from build123d import *

# Parameters (mm, degrees)
SKETCH2_R           = 13.75
BOSS_EXTRUDE1_DEPTH = 26.5
SKETCH3_R           = 2
BOSS_EXTRUDE2_DEPTH = 3.5
SKETCH4_R           = 1.25
CUT_EXTRUDE1_DEPTH  = 5
BOSS_EXTRUDE3_REACH = 39.959
SKETCH1_R           = 2
SKETCH5_R           = 1.25
CUT_EXTRUDE2_DEPTH  = 5


with BuildPart() as part:
    # Sketch2 → Boss-Extrude1 (new body)
    with BuildSketch(Plane(origin=(0, 2.6, 0), x_dir=(1, 0, 0), z_dir=(0, 1, 0))):
        with Locations(Location((0, 0, 0), (0, 0, 270))):
            Circle(SKETCH2_R)
    extrude(amount=BOSS_EXTRUDE1_DEPTH)

    # Sketch3 → Boss-Extrude2 (add)
    with BuildSketch(Plane(origin=(0, 29.1, 0), x_dir=(1, 0, 0), z_dir=(0, 1, 0))):
        with Locations(Location((0, 0, 0), (0, 0, 270))):
            Circle(SKETCH3_R)
    extrude(amount=BOSS_EXTRUDE2_DEPTH)

    # Sketch4 → Cut-Extrude1 (cut)
    with BuildSketch(Plane(origin=(0, 29.1, 0), x_dir=(1, 0, 0), z_dir=(0, 1, 0))):
        with Locations(Location((-6, 0, 0), (0, 0, 270))):
            Circle(SKETCH4_R)
        with Locations(Location((6, 0, 0), (0, 0, 270))):
            Circle(SKETCH4_R)
    extrude(amount=-CUT_EXTRUDE1_DEPTH, mode=Mode.SUBTRACT)

    # Sketch1 → Boss-Extrude3 (add, up to next)
    with BuildSketch(Plane(origin=(0, 0, 0), x_dir=(1, 0, 0), z_dir=(0, 1, 0)), mode=Mode.PRIVATE) as boss_extrude3_sk1:
        with Locations(Location((0, 0, 0), (0, 0, 270))):
            Circle(SKETCH1_R)
    boss_extrude3_tool1 = extrude(boss_extrude3_sk1.sketch, amount=BOSS_EXTRUDE3_REACH, mode=Mode.PRIVATE) - part.part
    add(boss_extrude3_tool1.solids().sort_by_distance((0, 0, 0))[0])

    # Sketch5 → Cut-Extrude2 (cut)
    with BuildSketch(Plane.XZ.offset(-2.6)):
        with Locations(Location((0, 9.000000034, 0), (0, 0, 270))):
            Circle(SKETCH5_R)
        with Locations(Location((0, -9.000000034, 0), (0, 0, 270))):
            Circle(SKETCH5_R)
        with Locations(Location((-9.5000001, 0, 0), (0, 0, 270))):
            Circle(SKETCH5_R)
        with Locations(Location((9.5, 0, 0), (0, 0, 270))):
            Circle(SKETCH5_R)
    extrude(amount=-CUT_EXTRUDE2_DEPTH, mode=Mode.SUBTRACT)


solid = part.part
Geometry: final body of the model. Coordinates: model frame, mm. A direction names the side the tool comes from. Round coordinates to 2 decimals unless told otherwise and drop trailing zeros. Write each loop counter-clockwise with the first axis right and the second up, starting at its lowest first coordinate (ties: lowest second). Pieces come first, ordered by that corner, then holes. Notation, with made-up numbers: M -1,3.5 L 53,3.5 A18 cw 53,13.5 Z; hole C -14,57.25 d1. An arc over 180 degrees is marked long. Write item = value, one per line.
Item 1: Pull-direction query (X, two-part tool) for faces 1 (the face through (-3, 29.1, 0)), 2 (the face through (4.78, 26.64, -0.27)), 3 (the face through (-2, 1, 0)), 4 (the face through (-6, 24.1, 0)); classes: pulls with the +X half, pulls with the -X half, needs draft (parallel to the pull), parting line crosses it, or undercut.
Findings:
face_1 = needs draft
face_2 = undercut
face_3 = parting line crosses it
face_4 = undercut
Item 2: Access query for faces 5 (the face through (-2, 31, 0)), 6 (the face through (0.05, 5.06, 10.25)), 7 (the face through (-12.2, 15.66, 6.34)). Directions: +Z, -Z, +X, -X, +Y, -Y. A direction counts if a zero-diameter tool reaches every point of the face in a straight line with its end or side. Return the directions, or none.
Findings:
face_5 = +Y
face_6 = -Y
face_7 = +Y, -Y
Item 3: Section query B-B on z = 0. Return loops of the section in (x, y).
Findings:
outline = M -13.75,2.6 L -10.75,2.6 L -10.75,7.6 L -8.25,7.6 L -8.25,2.6 L -2,2.6 L -2,0 L 2,0 L 2,2.6 L 8.25,2.6 L 8.25,7.6 L 10.75,7.6 L 10.75,2.6 L 13.75,2.6 L 13.75,29.1 L 7.25,29.1 L 7.25,24.1 L 4.75,24.1 L 4.75,29.1 L 2,29.1 L 2,32.6 L -2,32.6 L -2,29.1 L -4.75,29.1 L -4.75,24.1 L -7.25,24.1 L -7.25,29.1 L -13.75,29.1 Z
Item 4: Pin query (flat end, axial travel): P1, Ø4, axis at x = -5, z = 3, coming from the +Y side; P2, Ø1.5, axis at x = 6, z = 0, coming from the -Y side; P3, Ø0.8, axis at x = 5.5, z = 0, coming from the +Y side. Return the tip coordinate at first contact, or that it passes through.
Findings:
P1 = 29.1
P2 = 2.6
P3 = 24.1
Item 5: Section query D-D on y = 27. Return loops of the section in (x, z), then the cut area to 3 significant figures.
Findings:
outline = C 0,0 d27.5; hole C -6,0 d2.5; hole C 6,0 d2.5
area = 584 mm^2
Item 6: Section query C-C on x = 0. Return loops of the section in (y, z).
Findings:
outline = M 0,-2 L 2.6,-2 L 2.6,-7.75 L 7.6,-7.75 L 7.6,-10.25 L 2.6,-10.25 L 2.6,-13.75 L 29.1,-13.75 L 29.1,-2 L 32.6,-2 L 32.6,2 L 29.1,2 L 29.1,13.75 L 2.6,13.75 L 2.6,10.25 L 7.6,10.25 L 7.6,7.75 L 2.6,7.75 L 2.6,2 L 0,2 Z
Item 7: Section query A-A on y = 4.5. Return loops of the section in (x, z), then the cut area to 3 significant figures.
Findings:
outline = C 0,0 d27.5; hole C -9.5,0 d2.5; hole C 0,-9 d2.5; hole C 0,9 d2.5; hole C 9.5,0 d2.5
area = 574 mm^2
Item 8: Material intervals for line 1 along X through (y, z) = (6, 0); line 2 along Y through (x, z) = (-5, -12); line 3 along Z through (x, y) = (-9.5, 5.55), sorted ascending. Write a range as [from, to].
Findings:
line_1 = [-13.75, -10.75], [-8.25, 8.25], [10.75, 13.75]
line_2 = [2.6, 29.1]
line_3 = [-9.94, -1.25], [1.25, 9.94]
